from build123d import *

# Parameters (mm, degrees)
CYLINDER002_R          = 2.5
CYLINDER002_DEPTH      = 17
CYLINDER003_R          = 1.55
CYLINDER003_DEPTH      = 17
CYLINDER004_R          = 1.55
CYLINDER004_DEPTH      = 17
CYLINDER005_R          = 1.55
CYLINDER005_DEPTH      = 17
CYLINDER006_R          = 1.55
CYLINDER006_DEPTH      = 17
CYLINDER007_R          = 1.55
CYLINDER007_DEPTH      = 17
CYLINDER001_R          = 1.55
CYLINDER001_DEPTH      = 17
SKETCH019_R            = 8.4
PAD010_DEPTH           = 15
CUT009_PLACEMENT_ANGLE = 90


with BuildPart() as fibre002:
    # Cylinder002 → Cylinder002 (new body)
    with BuildSketch(Plane.XY):
        Circle(CYLINDER002_R)
    extrude(amount=CYLINDER002_DEPTH)


with BuildPart() as fibre003:
    # Cylinder003 → Cylinder003 (new body)
    with BuildSketch(Plane(origin=(1.5, -2.6, 0), x_dir=(1, 0, 0), z_dir=(0, 0, 1))):
        Circle(CYLINDER003_R)
    extrude(amount=CYLINDER003_DEPTH)


with BuildPart() as fibre004:
    # Cylinder004 → Cylinder004 (new body)
    with BuildSketch(Plane(origin=(3, 0, 0), x_dir=(1, 0, 0), z_dir=(0, 0, 1))):
        Circle(CYLINDER004_R)
    extrude(amount=CYLINDER004_DEPTH)


with BuildPart() as fibre005:
    # Cylinder005 → Cylinder005 (new body)
    with BuildSketch(Plane(origin=(-3, 0, 0), x_dir=(1, 0, 0), z_dir=(0, 0, 1))):
        Circle(CYLINDER005_R)
    extrude(amount=CYLINDER005_DEPTH)


with BuildPart() as fibre006:
    # Cylinder006 → Cylinder006 (new body)
    with BuildSketch(Plane(origin=(-1.5, 2.6, 0), x_dir=(1, 0, 0), z_dir=(0, 0, 1))):
        Circle(CYLINDER006_R)
    extrude(amount=CYLINDER006_DEPTH)


with BuildPart() as fibre007:
    # Cylinder007 → Cylinder007 (new body)
    with BuildSketch(Plane(origin=(-1.5, -2.6, 0), x_dir=(1, 0, 0), z_dir=(0, 0, 1))):
        Circle(CYLINDER007_R)
    extrude(amount=CYLINDER007_DEPTH)


with BuildPart() as fibres:
    # Cylinder001 → Cylinder001 (new body)
    with BuildSketch(Plane(origin=(1.5, 2.6, 0), x_dir=(1, 0, 0), z_dir=(0, 0, 1))):
        Circle(CYLINDER001_R)
    extrude(amount=CYLINDER001_DEPTH)

    # Fusion: union Fibre002, Fibre003, Fibre004, Fibre005, Fibre006, Fibre007
    add(fibre002.part)
    add(fibre003.part)
    add(fibre004.part)
    add(fibre005.part)
    add(fibre006.part)
    add(fibre007.part)


with BuildPart() as fibresholder:
    # Sketch019 → Pad010 (new body)
    with BuildSketch(Plane.XY):
        Circle(SKETCH019_R)
    extrude(amount=PAD010_DEPTH)

    # Cut009: cut Fibres
    add(fibres.part, mode=Mode.SUBTRACT)


with BuildPart() as fibresholder_1:
    # Cut009 placement: moved
    add(fibresholder.part.moved(Location((0, -53.7, 0))).rotate(Axis((0, -53.7, 0), (1, 0, 0)), CUT009_PLACEMENT_ANGLE))


solid = fibresholder_1.part
Geometry: final body of the model. Coordinates: model frame, mm. Coordinates: 2 decimals unless noted, no trailing zeros. Order: outer loops, then holes, each group sorted by start corner. A loop starts at its lowest first (then second) coordinate and runs counter-clockwise, first axis right, second up. Notation, with made-up numbers: (8.5, -24.75) - (25.5, -24.75) arc R11 cw to (25.5, -5.75) - close; hole circle Ø4 at (-12.5, -25). An arc over 180 degrees is marked (long way). Use one line per item in the form item = value.
1) Section C-C (x = -3.75). Return loops of the section in (y, z), then the cut area to 3 significant figures.
Solutions:
outline = (-68.7, -7.52) - (-53.7, -7.52) - (-53.7, -1.36) - (-68.7, -1.36) - close; (-68.7, 1.36) - (-53.7, 1.36) - (-53.7, 7.52) - (-68.7, 7.52) - close
area = 185 mm^2
2) Pin query (flat end, axial travel): pin 1 (2 mm diameter, centred on y = -57, z = -3.5, fed in from +X); pin 2 (1.9 mm diameter, centred on x = -1.5, z = 2.6, fed in from +Y); pin 3 (1.5 mm diameter, centred on x = 1, y = -57.5, fed in from -Z); pin 4 (4 mm diameter, centred on x = 1.5, z = -2.6, fed in from +Y). Return the tip coordinate at first contact, or that it passes through.
Solutions:
pin_1 = 8.02
pin_2 = through
pin_3 = -8.4
pin_4 = -53.7
3) Ray query, L1, parallel to X at y = -66, z = -3.25; L2, parallel to Z at x = -1.5, y = -58; L3, parallel to X at y = -64.5, z = 2.6. Return the intervals inside material, ascending.
Solutions:
L1 = -7.75 to -2.91, -0.09 to 0.09, 2.91 to 7.75
L2 = -8.26 to -4.15, 4.15 to 8.26
L3 = -7.99 to -3.05, 3.05 to 7.99
4) Section A-A (z = 0). Return loops of the section in (x, y), then the cut area to 4 significant figures.
Solutions:
outline = (-8.4, -68.7) - (-4.55, -68.7) - (-4.55, -53.7) - (-8.4, -53.7) - close; (4.55, -68.7) - (8.4, -68.7) - (8.4, -53.7) - (4.55, -53.7) - close
area = 115.5 mm^2
5) Section D-D (z = 4.75). Return loops of the section in (x, y), then the cut area to 3 significant figures.
Solutions:
outline = (-6.93, -68.7) - (6.93, -68.7) - (6.93, -53.7) - (-6.93, -53.7) - close
area = 208 mm^2
6) Section B-B (y = -62.75). Return loops of the section in (x, z).
Solutions:
outline = circle Ø16.8 at (0, 0); hole (-2.59, -1.49) arc R1.55 ccw (long way) to (0, -2.99) arc R1.55 ccw (long way) to (2.59, -1.49) arc R1.55 ccw (long way) to (2.59, 1.49) arc R1.55 ccw (long way) to (0, 2.99) arc R1.55 ccw (long way) to (-2.59, 1.49) arc R1.55 ccw (long way) to start
7) Mould query, pull axis X, two halves, no side actions, for faces 1 (the face through (0, -68.7, -4)), 2 (the face through (-2.31, -61.1, -3.92)), 3 (the face through (-1.09, -61.1, 8.33)). Classes: +X half, -X half, draft (parallel to the pull), parting line (faces both ways), or undercut.
Solutions:
face_1 = draft
face_2 = undercut
face_3 = parting line
